```python
from build123d import *

# Parameters (mm, degrees)
SKETCH1_W                                      = 401
SKETCH1_H                                      = 111
BOSS_EXTRUDE1_DEPTH                            = 13.5
SKETCH2_W                                      = 401
SKETCH2_H                                      = 111
SKETCH2_W_2                                    = 397
SKETCH2_H_2                                    = 107
CUT_EXTRUDE1_DEPTH                             = 1.5
FILLET1_R                                      = 6
FILLET2_R                                      = 4
CUT_EXTRUDE2_DEPTH                             = 8.5
SKETCH4_W                                      = 425.758885171
SKETCH4_H                                      = 132.096565748
CUT_EXTRUDE3_DEPTH                             = 1.5
CUT_EXTRUDE4_DEPTH                             = 8.5
CUT_EXTRUDE5_DEPTH                             = 8.5
FILLET3_R                                      = 3.175
CUT_EXTRUDE6_DEPTH                             = 0.375
CHAMFER1_SIZE                                  = 0.254
CUT_EXTRUDE7_DEPTH                             = 5
CUT_EXTRUDE7_DEPTH_BACK                        = 5
SKETCH8_W                                      = 16.017090682
SKETCH8_H                                      = 1.5
SKETCH9_R                                      = 37.5
CUT_EXTRUDE8_DEPTH                             = 10
BOSS_EXTRUDE4_DEPTH                            = 1
FILLET4_R                                      = 3.175
BOSS_EXTRUDE5_DEPTH                            = 7.5
CBORE_FOR_M2_SHCS2_D                           = 2.4
CBORE_FOR_M2_SHCS2_CBORE_D                     = 4.4
CBORE_FOR_M2_SHCS2_CBORE_DEPTH                 = 2.3
SKETCH33_W                                     = 427.456701586
SKETCH33_H                                     = 134.15369465
CUT_EXTRUDE9_DEPTH                             = 0.25
SKETCH37_R                                     = 45
BOSS_EXTRUDE6_DEPTH                            = 1.1
CSK_FOR_M4_FLAT_HEAD_MACHINE_SCREW1_AT_2_COUNT = 2
CSK_FOR_M4_FLAT_HEAD_MACHINE_SCREW1_AT_2_PITCH = 351
FILLET5_R                                      = 3.175
SKETCH40_W                                     = 472.271796357
SKETCH40_H                                     = 174.060638188
CUT_EXTRUDE10_DEPTH                            = 1.25


with BuildPart() as part:
    # Sketch1 → Boss-Extrude1 (new body)
    with BuildSketch(Plane(origin=(0, 0, 0), x_dir=(1, 0, 0), z_dir=(0, 1, 0))):
        with Locations((-200.5, 55.5)):
            Rectangle(SKETCH1_W, SKETCH1_H)
    extrude(amount=BOSS_EXTRUDE1_DEPTH)

    # Sketch2 → Cut-Extrude1 (cut)
    with BuildSketch(Plane(origin=(0, 13.5, 0), x_dir=(1, 0, 0), z_dir=(0, 1, 0))):
        with Locations((-200.5, 55.5)):
            Rectangle(SKETCH2_W, SKETCH2_H)
        with Locations((-200.5, 55.5)):
            Rectangle(SKETCH2_W_2, SKETCH2_H_2, mode=Mode.SUBTRACT)
    extrude(amount=-CUT_EXTRUDE1_DEPTH, mode=Mode.SUBTRACT)

    # Fillet1
    fillet1_edges = [part.edges().sort_by_distance(p)[0] for p in [
        (-2, 12.75, -2),
        (-399, 12.75, -2),
        (-399, 12.75, -109),
        (-2, 12.75, -109),
    ]]
    fillet(fillet1_edges, radius=FILLET1_R)

    # Fillet2
    fillet2_edges = [part.edges().sort_by_distance(p)[0] for p in [
        (0, 6, 0),
        (-401, 6, 0),
        (-401, 6, -111),
        (0, 6, -111),
    ]]
    fillet(fillet2_edges, radius=FILLET2_R)

    # Sketch3 → Cut-Extrude2 (cut)
    with BuildSketch(Plane(origin=(0, 13.5, 0), x_dir=(1, 0, 0), z_dir=(0, 1, 0))):
        with BuildLine():
            Line((-9.5, 6.5), (-391.5, 6.5))
            ThreePointArc((-391.5, 6.5), (-393.621320344, 7.378679656), (-394.5, 9.5))
            Line((-394.5, 9.5), (-394.5, 101.5))
            ThreePointArc((-394.5, 101.5), (-393.621320344, 103.621320344), (-391.5, 104.5))
            Line((-391.5, 104.5), (-9.5, 104.5))
            ThreePointArc((-9.5, 104.5), (-7.378679656, 103.621320344), (-6.5, 101.5))
            Line((-6.5, 101.5), (-6.5, 9.5))
            ThreePointArc((-6.5, 9.5), (-7.378679656, 7.378679656), (-9.5, 6.5))
        make_face()
    extrude(amount=-CUT_EXTRUDE2_DEPTH, mode=Mode.SUBTRACT)

    # Sketch4 → Cut-Extrude3 (cut)
    with BuildSketch(Plane.XZ):
        with Locations((-205.400573141, -53.58073678)):
            Rectangle(SKETCH4_W, SKETCH4_H)
    extrude(amount=-CUT_EXTRUDE3_DEPTH, mode=Mode.SUBTRACT)

    # Sketch5 → Cut-Extrude4 (cut)
    with BuildSketch(Plane(origin=(0, 13.5, 0), x_dir=(1, 0, 0), z_dir=(0, 1, 0))):
        with BuildLine():
            Line((-73.3928, 103.5), (-68.508545341, 108.058681888))
            ThreePointArc((-68.508545341, 108.058681888), (-67.403893551, 108.756177714), (-66.120419088, 109))
            Line((-66.120419088, 109), (-54.879580912, 109))
            ThreePointArc((-54.879580912, 109), (-53.596106449, 108.756177714), (-52.491454659, 108.058681888))
            Line((-52.491454659, 108.058681888), (-47.6072, 103.5))
            Line((-47.6072, 103.5), (-73.3928, 103.5))
        make_face()
    extrude(amount=-CUT_EXTRUDE4_DEPTH, mode=Mode.SUBTRACT)

    # Sketch6 → Cut-Extrude5 (cut)
    with BuildSketch(Plane.XY.offset(-109)):
        with BuildLine():
            Line((-63.900019088, 8.75), (-57.100019088, 8.75))
            ThreePointArc((-57.100019088, 8.75), (-56.216135611, 8.383883476), (-55.850019088, 7.5))
            Line((-55.850019088, 7.5), (-55.850019088, 6.25))
            ThreePointArc((-55.850019088, 6.25), (-56.216135611, 5.366116524), (-57.100019088, 5))
            Line((-57.100019088, 5), (-63.900019088, 5))
            ThreePointArc((-63.900019088, 5), (-64.783902564, 5.366116524), (-65.150019088, 6.25))
            Line((-65.150019088, 6.25), (-65.150019088, 7.5))
            ThreePointArc((-65.150019088, 7.5), (-64.783902564, 8.383883476), (-63.900019088, 8.75))
        make_face()
    extrude(amount=-CUT_EXTRUDE5_DEPTH, mode=Mode.SUBTRACT)

    # Fillet3
    fillet3_edges = [part.edges().sort_by_distance(p)[0] for p in [
        (-1.171572875, 1.5, -109.828427125),
        (-401, 1.5, -55.5),
        (-200.5, 1.5, -111),
        (0, 1.5, -55.5),
        (-200.5, 1.5, 0),
        (-399.828427125, 1.5, -1.171572875),
        (-1.171572875, 1.5, -1.171572875),
        (-399.828427125, 1.5, -109.828427125),
    ]]
    fillet(fillet3_edges, radius=FILLET3_R)

    # Sketch7 → Cut-Extrude6 (cut)
    with BuildSketch(Plane(origin=(0, 0, -111), x_dir=(-1, 0, 0), z_dir=(0, 0, -1))):
        with BuildLine():
            Line((56.675019088, 11.125), (64.325019088, 11.125))
            ThreePointArc((64.325019088, 11.125), (66.570083118, 10.19506403), (67.500019088, 7.95))
            Line((67.500019088, 7.95), (67.500019088, 1.125))
            Line((67.500019088, 1.125), (53.500019088, 1.125))
            Line((53.500019088, 1.125), (53.500019088, 7.95))
            ThreePointArc((53.500019088, 7.95), (54.429955058, 10.19506403), (56.675019088, 11.125))
        make_face()
    extrude(amount=-CUT_EXTRUDE6_DEPTH, mode=Mode.SUBTRACT)

    # Chamfer1
    chamfer1_edges = [part.edges().sort_by_distance(p)[0] for p in [
        (-56.216135611, 5.366116524, -110.625),
        (-55.850019088, 6.875, -110.625),
        (-56.216135611, 8.383883476, -110.625),
        (-60.500019088, 8.75, -110.625),
        (-64.783902564, 8.383883476, -110.625),
        (-65.150019088, 6.875, -110.625),
        (-64.783902564, 5.366116524, -110.625),
        (-60.500019088, 5, -110.625),
    ]]
    chamfer(chamfer1_edges, length=CHAMFER1_SIZE)

    # Sketch8 → Cut-Extrude7 (cut, two sides: drawn at the far end of the back side and taken through both)
    with BuildSketch(Plane(origin=(0, 0, -109), x_dir=(-1, 0, 0), z_dir=(0, 0, -1)).offset(-CUT_EXTRUDE7_DEPTH_BACK)):
        with Locations((60.5, 12.75)):
            Rectangle(SKETCH8_W, SKETCH8_H)
    extrude(amount=CUT_EXTRUDE7_DEPTH + CUT_EXTRUDE7_DEPTH_BACK, mode=Mode.SUBTRACT)

    # Sketch9 → Cut-Extrude8 (cut)
    with BuildSketch(Plane.XZ.offset(-1.5)):
        with Locations(Location((-200.5, -55.5, 0), (0, 0, 270))):
            Circle(SKETCH9_R)
    extrude(amount=-CUT_EXTRUDE8_DEPTH, mode=Mode.SUBTRACT)

    # Sketch25 → Boss-Extrude4 (add)
    with BuildSketch(Plane(origin=(0, 5, 0), x_dir=(1, 0, 0), z_dir=(0, 1, 0))):
        with BuildLine():
            Line((-138.370726122, 104.5), (-132.379273878, 104.5))
            ThreePointArc((-132.379273878, 104.5), (-135.375, 102.425), (-138.370726122, 104.5))
        make_face()
        with BuildLine():
            Line((-268.620726122, 104.5), (-262.629273878, 104.5))
            ThreePointArc((-262.629273878, 104.5), (-265.625, 102.425), (-268.620726122, 104.5))
        make_face()
        with BuildLine():
            Line((-138.370726122, 6.5), (-132.379273878, 6.5))
            ThreePointArc((-132.379273878, 6.5), (-135.375, 8.575), (-138.370726122, 6.5))
        make_face()
        with BuildLine():
            Line((-268.620726122, 6.5), (-262.629273878, 6.5))
            ThreePointArc((-262.629273878, 6.5), (-265.625, 8.575), (-268.620726122, 6.5))
        make_face()
    extrude(amount=BOSS_EXTRUDE4_DEPTH)

    # Fillet4
    fillet4_edges = [part.edges().sort_by_distance(p)[0] for p in [
        (-268.620726122, 5.5, -104.5),
        (-262.629273878, 5.5, -104.5),
        (-138.370726122, 5.5, -104.5),
        (-132.379273878, 5.5, -104.5),
        (-132.379273878, 5.5, -6.5),
        (-138.370726122, 5.5, -6.5),
        (-262.629273878, 5.5, -6.5),
        (-268.620726122, 5.5, -6.5),
    ]]
    fillet(fillet4_edges, radius=FILLET4_R)

    # Sketch27 → Boss-Extrude5 (add)
    with BuildSketch(Plane(origin=(0, 6, 0), x_dir=(1, 0, 0), z_dir=(0, 1, 0))):
        with BuildLine():
            Line((-267.427775638, 104.5), (-263.822224362, 104.5))
            ThreePointArc((-263.822224362, 104.5), (-265.625, 103.5), (-267.427775638, 104.5))
        make_face()
        with BuildLine():
            Line((-137.177775638, 104.5), (-133.572224362, 104.5))
            ThreePointArc((-133.572224362, 104.5), (-135.375, 103.5), (-137.177775638, 104.5))
        make_face()
        with BuildLine():
            Line((-137.177775638, 6.5), (-133.572224362, 6.5))
            ThreePointArc((-133.572224362, 6.5), (-135.375, 7.5), (-137.177775638, 6.5))
        make_face()
        with BuildLine():
            Line((-267.427775638, 6.5), (-263.822224362, 6.5))
            ThreePointArc((-263.822224362, 6.5), (-265.625, 7.5), (-267.427775638, 6.5))
        make_face()
    extrude(amount=BOSS_EXTRUDE5_DEPTH)

    # CBORE for M2 SHCS2 (through all)
    with Locations(Plane(origin=(-5.375, 1.5, -105.625), x_dir=(0, 0, -1), z_dir=(0, -1, 0))):
        with Locations((0, 0), (0, -130), (0, -260.25), (0, -390.25), (-100.25, -390.25), (-100.25, -260.25), (-100.25, -130), (-100.25, 0)):
            CounterBoreHole(CBORE_FOR_M2_SHCS2_D / 2, CBORE_FOR_M2_SHCS2_CBORE_D / 2, CBORE_FOR_M2_SHCS2_CBORE_DEPTH)

    # Sketch33 → Cut-Extrude9 (cut)
    with BuildSketch(Plane(origin=(0, 13.5, 0), x_dir=(1, 0, 0), z_dir=(0, 1, 0))):
        with Locations((-199.55079933, 53.126998326)):
            Rectangle(SKETCH33_W, SKETCH33_H)
    extrude(amount=-CUT_EXTRUDE9_DEPTH, mode=Mode.SUBTRACT)

    # Sketch37 → Boss-Extrude6 (add)
    with BuildSketch(Plane(origin=(0, 5, 0), x_dir=(1, 0, 0), z_dir=(0, 1, 0))):
        with Locations((-200.5, 55.5)):
            Circle(SKETCH37_R)
    extrude(amount=-BOSS_EXTRUDE6_DEPTH)

    # Sketch38 → CSK for M4 Flat Head Machine Screw1 (revolve, cut)
    with BuildSketch(Plane(origin=(-376, 5, -86), x_dir=(0, 0, 1), z_dir=(1, 0, 0))):
        Polygon((0, 0), (0, 3.5), (2.25, 3.5), (2.25, 2.75), (5, 0), align=None)
    csk_for_m4_flat_head_machine_screw1 = revolve(axis=Axis((-376, 11.35, -86), (0, -1, 0)), mode=Mode.SUBTRACT)

    # CSK for M4 Flat Head Machine Screw1 at 2: CSK for M4 Flat Head Machine Screw1 ×2
    with Locations(*[(i * CSK_FOR_M4_FLAT_HEAD_MACHINE_SCREW1_AT_2_PITCH, 0, 0) for i in range(1, CSK_FOR_M4_FLAT_HEAD_MACHINE_SCREW1_AT_2_COUNT)]):
        add(csk_for_m4_flat_head_machine_screw1, mode=Mode.SUBTRACT)

    # Fillet5
    fillet5_edges = [part.edges().sort_by_distance(p)[0] for p in [
        (-263.822224362, 9.625, -6.5),
        (-267.427775638, 9.625, -6.5),
        (-133.572224362, 9.625, -6.5),
        (-137.177775638, 9.625, -6.5),
        (-137.177775638, 9.625, -104.5),
        (-133.572224362, 9.625, -104.5),
        (-267.427775638, 9.625, -104.5),
        (-263.822224362, 9.625, -104.5),
    ]]
    fillet(fillet5_edges, radius=FILLET5_R)

    # Sketch40 → Cut-Extrude10 (cut)
    with BuildSketch(Plane(origin=(0, 13.25, 0), x_dir=(1, 0, 0), z_dir=(0, 1, 0))):
        with Locations((-179.677600421, 43.410464589)):
            Rectangle(SKETCH40_W, SKETCH40_H)
        with BuildLine():
            Line((-52.491454659, 108.875), (-8, 108.875))
            ThreePointArc((-8, 108.875), (-3.845747661, 107.154252339), (-2.125, 103))
            Line((-2.125, 103), (-2.125, 8))
            ThreePointArc((-2.125, 8), (-3.845747661, 3.845747661), (-8, 2.125))
            Line((-8, 2.125), (-393, 2.125))
            ThreePointArc((-393, 2.125), (-397.154252339, 3.845747661), (-398.875, 8))
            Line((-398.875, 8), (-398.875, 103))
            ThreePointArc((-398.875, 103), (-397.154252339, 107.154252339), (-393, 108.875))
            Line((-393, 108.875), (-52.491454659, 108.875))
        make_face(mode=Mode.SUBTRACT)
    extrude(amount=-CUT_EXTRUDE10_DEPTH, mode=Mode.SUBTRACT)


solid = part.part
```
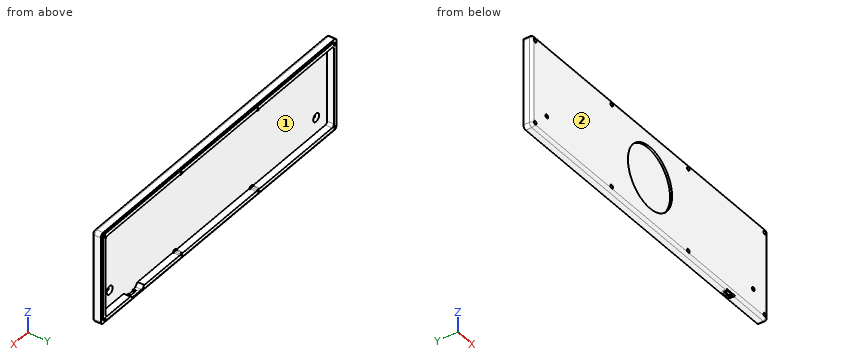
CAD build for the part. Positions are in the model's coordinates, mm. Face numbers are marked on the shaded views. Round coordinates to 2 decimals unless told otherwise and drop trailing zeros. Write each loop counter-clockwise with the first axis right and the second up, starting at its lowest first coordinate (ties: lowest second). Pieces come first, ordered by that corner, then holes. Notation, with made-up numbers: (-12.75, -9) -> (36.25, -9) arc R22 ccw to (36.25, 19) -> close; hole circle Ø11 at (3.25, 29). An arc over 180 degrees is marked (long way). Answer in a Markdown table with one row per item. Add a question column.
Item 1: Mould opens along Z. For the marked faces 1 and 2 say: pulls with the +Z half, pulls with the -Z half, needs draft (parallel to the pull), parting line crosses it, or undercut.
Item 2: Saw through at B-B, the plane z = -55.5. Write the cut outline in (x, y) (3 decimals).
Item 3: Drop flat-ended pins along their axis: pin 1 Ø6 at (x, z) = (-210.5, -14.5) entering from +Y; pin 2 Ø3 at (x, y) = (-143, 2.5) entering from -Z; pin 3 Ø1.4 at (x, y) = (-39, 13) entering from -Z (3 decimals). Give the stop position or say it passes through.
Item 4: Saw through at A-A, the plane x = -200.5. Write the cut outline in (y, z) (3 decimals), then the cut area to 3 significant figures.
Item 5: Saw through at C-C, the plane x = -281.5. Write the cut outline in (y, z) (3 decimals).
Item 6: Drill centre lines: line 1 (X direction, y = 12.75, z = -90) (3 decimals); line 2 (X direction, y = 6.5, z = -29.5); line 3 (Z direction, x = -285, y = 11.5). Where is each one in solid material? Low to high. Write a range as from..to.
Findings below:
| question | item | result |
|---|---|---|
| 1 | face 1 | undercut |
| 1 | face 2 | needs draft |
| 2 | outline | (-401, 4.675) arc R3.175 ccw to (-397.825, 1.5) -> (-238, 1.5) -> (-238, 3.9) -> (-163, 3.9) -> (-163, 1.5) -> (-3.175, 1.5) arc R3.175 ccw to (0, 4.675) -> (0, 12) -> (-2.125, 12) -> (-2.125, 13.25) -> (-6.5, 13.25) -> (-6.5, 5) -> (-394.5, 5) -> (-394.5, 13.25) -> (-398.875, 13.25) -> (-398.875, 12) -> (-401, 12) -> close |
| 3 | pin 1 | stops at y = 5 |
| 3 | pin 2 | stops at z = -110.93 |
| 3 | pin 3 | stops at z = -108.875 |
| 4 | outline | (1.5, -107.825) arc R3.175 ccw to (4.675, -111) -> (12, -111) -> (12, -108.875) -> (13.25, -108.875) -> (13.25, -104.5) -> (5, -104.5) -> (5, -6.5) -> (13.25, -6.5) -> (13.25, -2.125) -> (12, -2.125) -> (12, 0) -> (4.675, 0) arc R3.175 ccw to (1.5, -3.175) -> (1.5, -18) -> (3.9, -18) -> (3.9, -93) -> (1.5, -93) -> close |
| 4 | area | 306 mm^2 |
| 5 | outline | (1.5, -107.825) arc R3.175 ccw to (4.675, -111) -> (12, -111) -> (12, -108.875) -> (13.25, -108.875) -> (13.25, -104.5) -> (5, -104.5) -> (5, -6.5) -> (13.25, -6.5) -> (13.25, -2.125) -> (12, -2.125) -> (12, 0) -> (4.675, 0) arc R3.175 ccw to (1.5, -3.175) -> close |
| 6 | line 1 | x = -398.875..-394.5, -6.5..-2.125 |
| 6 | line 2 | x = -401..-394.5, -6.5..0 |
| 6 | line 3 | z = -111..-104.5, -6.5..0 |
